```python
from build123d import *

# Parameters (mm, degrees)
F1_DEPTH = 2
F4_DEPTH = 20


with BuildPart() as f1:
    # F0 (on Top) → F1 (new body)
    with BuildSketch(Plane.XY):
        Polygon((30, 40.5), (0, 40.5), (0, 20.5), (22, 20.5), (22, 0), (30, 0), align=None)
    extrude(amount=F1_DEPTH)

    # F3 (on offset) → F4 (join, through all)
    with BuildSketch(Plane(origin=(0, 40.5, 0), x_dir=(-1, 0, 0), z_dir=(0, 1, 0))):
        with BuildLine():
            ThreePointArc((0, 0), (3.5, -3.5), (7, 0))
            ThreePointArc((7, 0), (4.8682335874, 3.221480537), (1.0697503713, 2.5187073554))
            ThreePointArc((1.0697503713, 2.5187073554), (0.278519463, 1.3682335874), (0, 0))
        make_face()
        with BuildLine():
            ThreePointArc((0, 0), (0.278519463, 1.3682335874), (1.0697503713, 2.5187073554))
            add(Edge.make_bspline(
                [(1.0697503713, 2.5187073554), (0.8128216168, 2.2708020127), (0.3570286317, 2), (0, 2)],
                knots=[0, 0, 0, 0, 1.1888747527, 1.1888747527, 1.1888747527, 1.1888747527], degree=3))
            Line((0, 2), (0, 0))
        make_face()
    extrude(amount=-F4_DEPTH)

    # F5: F1 across plane


with BuildPart() as f1_1:
    add(f1.part)
    add(f1.part.mirror(Plane.XZ))


solid = f1_1.part
```
Can you work these out from the model? Positions are in its coordinate system, mm. A direction names the side the tool comes from. Round coordinates to 2 decimals unless told otherwise and drop trailing zeros. Loops run counter-clockwise (first coordinate to the right, second up) from the corner with the lowest first, then second, coordinate; pieces in that order, holes last. Notation, with made-up numbers: (81, 85.5) -> (114, 85.5) arc R18 ccw to (114, 102.5) -> close; hole circle Ø9 at (40.5, 80). An arc over 180 degrees is marked (long way). Answer in a Markdown table with one row per item.
Item 1: Suppose I cut it at A-A, the plane x = 15.5. List the corners of the cut face in (y, z) for me.
Answer block:
| item | result |
|---|---|
| outline | (-40.5, 0) -> (-20.5, 0) -> (-20.5, 2) -> (-40.5, 2) -> close; (20.5, 0) -> (40.5, 0) -> (40.5, 2) -> (20.5, 2) -> close |
Item 2: Suppose I cut it at B-B, the plane z = -1. List the corners of the cut face in (x, y) for me, plus the area to 3 significant figures.
Answer block:
| item | result |
|---|---|
| outline | (-6.85, -40.5) -> (-0.15, -40.5) -> (-0.15, -20.5) -> (-6.85, -20.5) -> close; (-6.85, 20.5) -> (-0.15, 20.5) -> (-0.15, 40.5) -> (-6.85, 40.5) -> close |
| area | 268 mm² |
Item 3: We'd pull the mould along Y, two halves only. Please class faces 4 (the flat face through (22, 0, 1)), 5 (the flat face through (8, 40.5, 1)), 6 (the flat face through (25, -1, 0)): released by +Y, released by -Y, zero draft, split by the parting line, or undercut.
Answer block:
| item | result |
|---|---|
| face 4 | undercut |
| face 5 | released by +Y |
| face 6 | zero draft |
Item 4: Will these pins go through, and if not, where does the flat tip stop? P1, Ø1.5, axis at x = 11.5, y = -21.5, coming from the +Z side; P2, Ø1.6, axis at y = -10, z = 1, coming from the -X side.
Answer block:
| item | result |
|---|---|
| P1 | z = 2 |
| P2 | x = 22 |
Item 5: If I drill on probe 1 along Y at (x, z) = (-2, -1.5); probe 2 along Z at (x, y) = (7.5, 36.5); probe 3 along X at (y, z) = (-19, 1.75), over which ranges is the centre line in solid material (lowest first)?
Answer block:
| item | result |
|---|---|
| probe 1 | -40.5 to -20.5, 20.5 to 40.5 |
| probe 2 | 0 to 2 |
| probe 3 | 22 to 30 |
Item 6: Suppose I cut it at C-C, the plane y = 13. List the corners of the cut face in (x, z) for me, plus the area to 3 significant figures.
Answer block:
| item | result |
|---|---|
| outline | (22, 0) -> (30, 0) -> (30, 2) -> (22, 2) -> close |
| area | 16.0 mm² |
Item 7: On a 3-axis mill with a long thin cutter (end or side, diameter ignored), from which of +Z, -Z, +X, -X, +Y, -Y can I reach the whole of each face in a straight line? I mean faces 1 (the flat face through (25, -1, 2)), 2 (the flat face through (8, -40.5, 1)), 3 (the flat face through (4, -20.5, 1)). Say none if no direction works.
Answer block:
| item | result |
|---|---|
| face 1 | +Z, +X, +Y, -Y |
| face 2 | +Z, -Z, +X, -X, -Y |
| face 3 | +Z, -Z, -X |
